Geometry: final body of the model. Coordinates: model frame, mm. Face numbers are marked on the shaded views. Coordinates: 2 decimals unless noted, no trailing zeros. Order: outer loops, then holes, each group sorted by start corner. A loop starts at its lowest first (then second) coordinate and runs counter-clockwise, first axis right, second up. Notation, with made-up numbers: M 78.25,56 L 118.25,56 A22 cw 118.25,91 Z; hole C 3.5,-23 d8. An arc over 180 degrees is marked long. One line per question, with ' | ' between items.
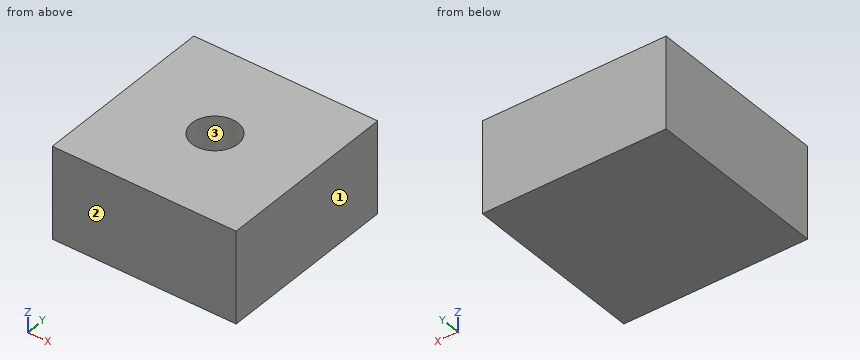
from build123d import *

# Parameters (mm, degrees)
SKETCH_1_W          = 20
SKETCH_1_H          = 20
BASEBOX_DEPTH       = 10
HOLE_WIZARD_1_D     = 5
HOLE_WIZARD_1_DEPTH = 5


with BuildPart() as part:
    # 草图1 → BaseBox (new body)
    with BuildSketch(Plane.XY):
        with Locations((10, 10)):
            Rectangle(SKETCH_1_W, SKETCH_1_H)
    extrude(amount=BASEBOX_DEPTH)

    # 孔1
    with Locations(Plane.XY.offset(10)):
        with Locations((9.986487375, 10.014305599)):
            Hole(HOLE_WIZARD_1_D / 2, depth=HOLE_WIZARD_1_DEPTH)


solid = part.part
1. Section B-B, the plane x = 11.5. Output: boundary loops of the cut face in (y, z).
Response values:
outline: M 0,0 L 20,0 L 20,10 L 12,10 L 12,5 L 8.02,5 L 8.02,10 L 0,10 Z
2. Material intervals for line 1 (Z direction, x = 8.5, y = 9.25); line 2 (Y direction, x = 10.5, z = 9.5); line 3 (Y direction, x = 8.5, z = 9.75), sorted ascending. Write a range as [from, to].
Response values:
line 1: z = [0, 5] | line 2: y = [0, 7.57], [12.46, 20] | line 3: y = [0, 8], [12.02, 20]
3. Draft query along X for the marked faces 1, 2 and 3. Return one class per face: pulls with the +X half, pulls with the -X half, needs draft (parallel to the pull), parting line crosses it, or undercut.
Response values:
face 1: pulls with the +X half | face 2: needs draft | face 3: undercut
4. Section A-A, the plane y = 9.25. Output: boundary loops of the cut face in (x, z), and give its area (3 significant figures).
Response values:
outline: M 0,0 L 20,0 L 20,10 L 12.37,10 L 12.37,5 L 7.61,5 L 7.61,10 L 0,10 Z | area: 176 mm^2
5. Section C-C, the plane z = 7.5. Output: boundary loops of the cut face in (x, y).
Response values:
outline: M 0,0 L 20,0 L 20,20 L 0,20 Z; hole C 9.99,10.01 d5
